```python
from build123d import *

# Parameters (mm, degrees)
BOSS_EXTRUDE1_DEPTH = 2.5
FILLET1_R           = 0.4
FILLET2_R           = 0.1


with BuildPart() as part:
    # Sketch2 → Boss-Extrude1 (new body)
    with BuildSketch(Plane.XY):
        with BuildLine():
            Line((0.4, 16.7), (6.932774682, 16.7))
            Line((6.932774682, 16.7), (-0.481596575, 12.925))
            Line((-0.481596575, 12.925), (7.718403425, 8.75))
            Line((7.718403425, 8.75), (-0.481596575, 4.575))
            Line((-0.481596575, 4.575), (6.932774682, 0.8))
            Line((6.932774682, 0.8), (0.4, 0.8))
            ThreePointArc((0.4, 0.8), (0, 0.4), (0.4, 0))
            Line((0.4, 0), (10.267225318, 0))
            Line((10.267225318, 0), (1.281596575, 4.575))
            Line((1.281596575, 4.575), (9.481596575, 8.75))
            Line((9.481596575, 8.75), (1.281596575, 12.925))
            Line((1.281596575, 12.925), (10.267225318, 17.5))
            Line((10.267225318, 17.5), (0.4, 17.5))
            ThreePointArc((0.4, 17.5), (0, 17.1), (0.4, 16.7))
        make_face()
    extrude(amount=BOSS_EXTRUDE1_DEPTH)

    # Fillet1
    fillet1_edges = [part.edges().sort_by_distance(p)[0] for p in [
        (10.267225318, 17.5, 1.25),
        (9.481596575, 8.75, 1.25),
        (10.267225318, 0, 1.25),
        (-0.481596575, 4.575, 1.25),
        (-0.481596575, 12.925, 1.25),
    ]]
    fillet(fillet1_edges, radius=FILLET1_R)

    # Fillet2
    fillet2_edges = [part.edges().sort_by_distance(p)[0] for p in [
        (1.281596575, 12.925, 1.25),
        (1.281596575, 4.575, 1.25),
        (6.932774682, 0.8, 1.25),
        (7.718403425, 8.75, 1.25),
        (6.932774682, 16.7, 1.25),
    ]]
    fillet(fillet2_edges, radius=FILLET2_R)


solid = part.part
```
The listing builds one solid part. Answer for the finished solid, in the listing's coordinates (mm). A direction names the side the tool comes from. Coordinates: 2 decimals unless noted, no trailing zeros. Order: outer loops, then holes, each group sorted by start corner. A loop starts at its lowest first (then second) coordinate and runs counter-clockwise, first axis right, second up. Notation, with made-up numbers: M -27,38 L -1,38 A26 ccw -1,71 Z; hole C 83.25,-36.75 d11. An arc over 180 degrees is marked long. Answer as a JSON object with one key per item and string values. Group by question number.
1. A flat-ended cylindrical pin translates along its axis: P1, Ø1.5, axis at y = 6, z = 1, coming from the +X side. Find the tip coordinate at first contact, or state that the pin passes through.
2. Section B-B on z = 0.6 is taken. Write down the section's boundary in (x, y) (3 decimals), then the cut area to 3 significant figures.
3. Section A-A on x = 2.5 is taken. Write down the section's boundary in (y, z), then the cut area to 3 significant figures.
4. Determine the mould class of faces 1 (the flat face through (4, 0, 1)), 2 (the flat face through (5, 17.5, 1)), 3 (the flat face through (5.5, 10.1, 2.5)), 4 (the flat face through (3.4, 14.9, 1.2)) for opening direction Y: released by +Y, released by -Y, zero draft, split by the parting line, or undercut.
5. Straight lines are drawn through the part: line 1 (Y direction, x = 2.75, z = 2); line 2 (Y direction, x = 0.5, z = 1.05); line 3 (Y direction, x = 7.5, z = 0.65). For each, find the intervals that lie inside material, in ascending order.
6. Section D-D on y = 2 is taken. Write down the section's boundary in (x, z).
7. Section C-C on x = 8 is taken. Write down the section's boundary in (y, z), then the cut area to 3 significant figures.
8. A tool of negligible diameter and unlimited length cuts with its end or side. For faces 5 (the flat face through (5.068, 6.503, 1.232)), 6 (the flat face through (3, 16.7, 1)), 7 (the flat face through (5.5, 10.1, 0)), from which of +Z, -Z, +X, -X, +Y, -Y can it reach the whole face along a straight path? Write none if from no direction.
Values follow:
{
 "1": {"P1": "x = 5.55"},
 "2": {"outline": "M 0.219,4.219 L 6.561,0.989 A0.1 cw 6.516,0.8 L 0.4,0.8 A0.4 ccw 0.4,0 L 8.6,0 A0.4 ccw 8.781,0.756 L 1.457,4.486 A0.1 cw 1.457,4.664 L 8.781,8.394 A0.4 ccw 8.781,9.106 L 1.457,12.836 A0.1 cw 1.457,13.014 L 8.781,16.744 A0.4 ccw 8.6,17.5 L 0.4,17.5 A0.4 ccw 0.4,16.7 L 6.516,16.7 A0.1 cw 6.561,16.511 L 0.219,13.281 A0.4 ccw 0.219,12.569 L 7.543,8.839 A0.1 cw 7.543,8.661 L 0.219,4.931 A0.4 ccw Z", "area": "41.8 mm2"},
 "3": {"outline": "M 0,0 L 0.8,0 L 0.8,2.5 L 0,2.5 Z; M 3.06,0 L 3.95,0 L 3.95,2.5 L 3.06,2.5 Z; M 5.2,0 L 6.09,0 L 6.09,2.5 L 5.2,2.5 Z; M 11.41,0 L 12.3,0 L 12.3,2.5 L 11.41,2.5 Z; M 13.55,0 L 14.44,0 L 14.44,2.5 L 13.55,2.5 Z; M 16.7,0 L 17.5,0 L 17.5,2.5 L 16.7,2.5 Z", "area": "13.0 mm2"},
 "4": {"face 1": "released by -Y", "face 2": "released by +Y", "face 3": "zero draft", "face 4": "undercut"},
 "5": {"line 1": "0 to 0.8, 2.93 to 3.83, 5.32 to 6.22, 11.28 to 12.18, 13.67 to 14.57, 16.7 to 17.5", "line 2": "0 to 0.8, 4.08 to 5.07, 12.43 to 13.42, 16.7 to 17.5", "line 3": "0 to 1.41, 7.74 to 8.64, 8.86 to 9.76, 16.09 to 17.5"},
 "6": {"outline": "M 4.58,0 L 6.34,0 L 6.34,2.5 L 4.58,2.5 Z"},
 "7": {"outline": "M 0,0 L 1.15,0 L 1.15,2.5 L 0,2.5 Z; M 8,0 L 9.5,0 L 9.5,2.5 L 8,2.5 Z; M 16.35,0 L 17.5,0 L 17.5,2.5 L 16.35,2.5 Z", "area": "9.54 mm2"},
 "8": {"face 5": "+Z, -Z, +X", "face 6": "+Z, -Z, -X", "face 7": "-Z, +X, -X, +Y, -Y"}
}
